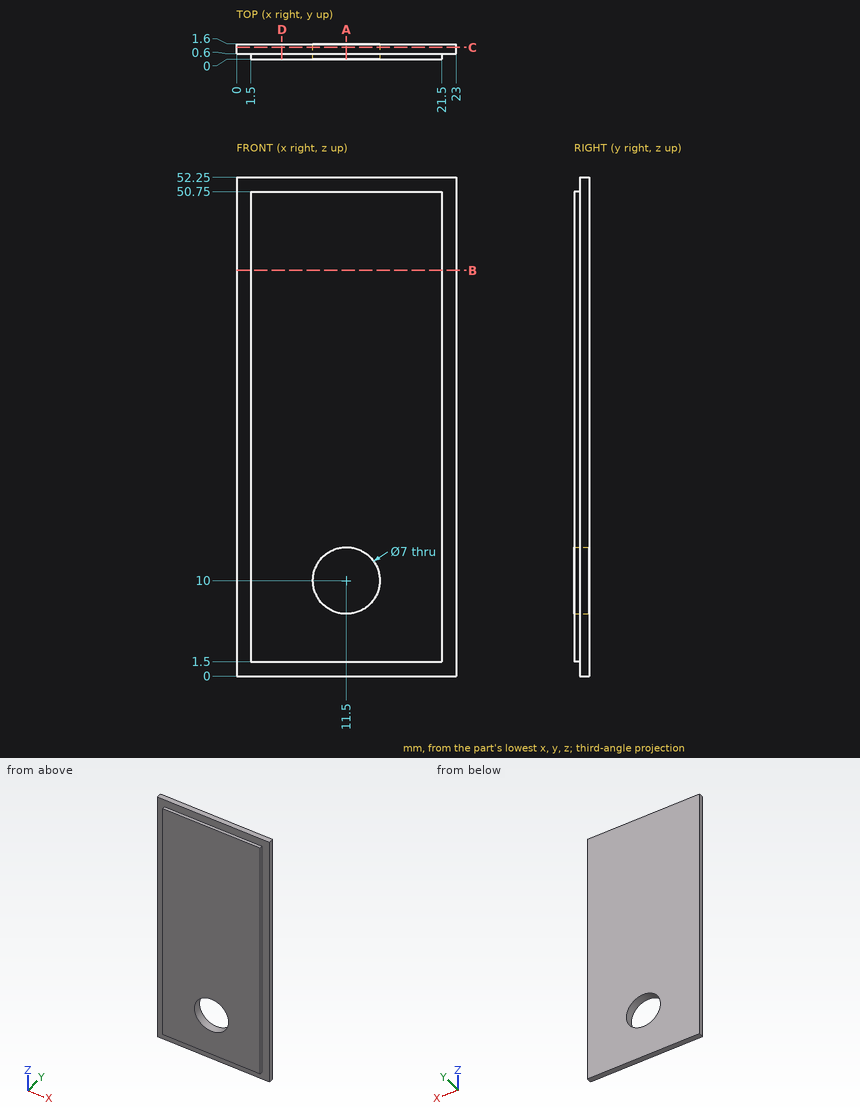
Geometry: see drawing. Coordinates: mm, zero at the bounding-box minimum. Round coordinates to 2 decimals unless told otherwise and drop trailing zeros. Order: outer loops, then holes, each group sorted by start corner. A loop starts at its lowest first (then second) coordinate and runs counter-clockwise, first axis right, second up. Notation, with made-up numbers: (0, 82) - (56, 82) arc R25 ccw to (56, 98) - close; hole circle Ø2 at (53, 47.5). An arc over 180 degrees is marked (long way). Use a Markdown table: item, result. Add a question column.
1. Section query D-D (x = 4.75). Return the cut outline in (y, z), then the cut area to 3 significant figures.
2. First-contact query: pin 1 (4 mm diameter, centred on x = 11.5, z = 10, fed in from +Y); pin 2 (0.5 mm diameter, centred on y = 0, z = 34, fed in from +X). Flat tips, straight axial feed; report the tip coordinate or a pass-through.
3. Line query: probe 1 along Z at (x, y) = (11.5, 0.55); probe 2 along Z at (x, y) = (11.5, 0.85); probe 3 along X at (y, z) = (0.45, 10). Output: solid intervals per line, ascending.
4. Section query A-A (x = 11.5). Return the cut outline in (y, z).
5. Section query C-C (y = 1.25). Return the cut outline in (x, z).
6. Section query B-B (z = 42.5). Return the cut outline in (x, y).
Derived:
| question | item | result |
|---|---|---|
| 1 | outline | (0, 1.5) - (0.6, 1.5) - (0.6, 0) - (1.6, 0) - (1.6, 52.25) - (0.6, 52.25) - (0.6, 50.75) - (0, 50.75) - close |
| 1 | area | 81.8 mm2 |
| 2 | pin 1 | through |
| 2 | pin 2 | x = 21.5 |
| 3 | probe 1 | 1.5 to 6.5, 13.5 to 50.75 |
| 3 | probe 2 | 0 to 6.5, 13.5 to 52.25 |
| 3 | probe 3 | 1.5 to 8, 15 to 21.5 |
| 4 | outline | (0, 1.5) - (0.6, 1.5) - (0.6, 0) - (1.6, 0) - (1.6, 6.5) - (0, 6.5) - close; (0, 13.5) - (1.6, 13.5) - (1.6, 52.25) - (0.6, 52.25) - (0.6, 50.75) - (0, 50.75) - close |
| 5 | outline | (0, 0) - (23, 0) - (23, 52.25) - (0, 52.25) - close; hole circle Ø7 at (11.5, 10) |
| 6 | outline | (0, 0.6) - (1.5, 0.6) - (1.5, 0) - (21.5, 0) - (21.5, 0.6) - (23, 0.6) - (23, 1.6) - (0, 1.6) - close |
